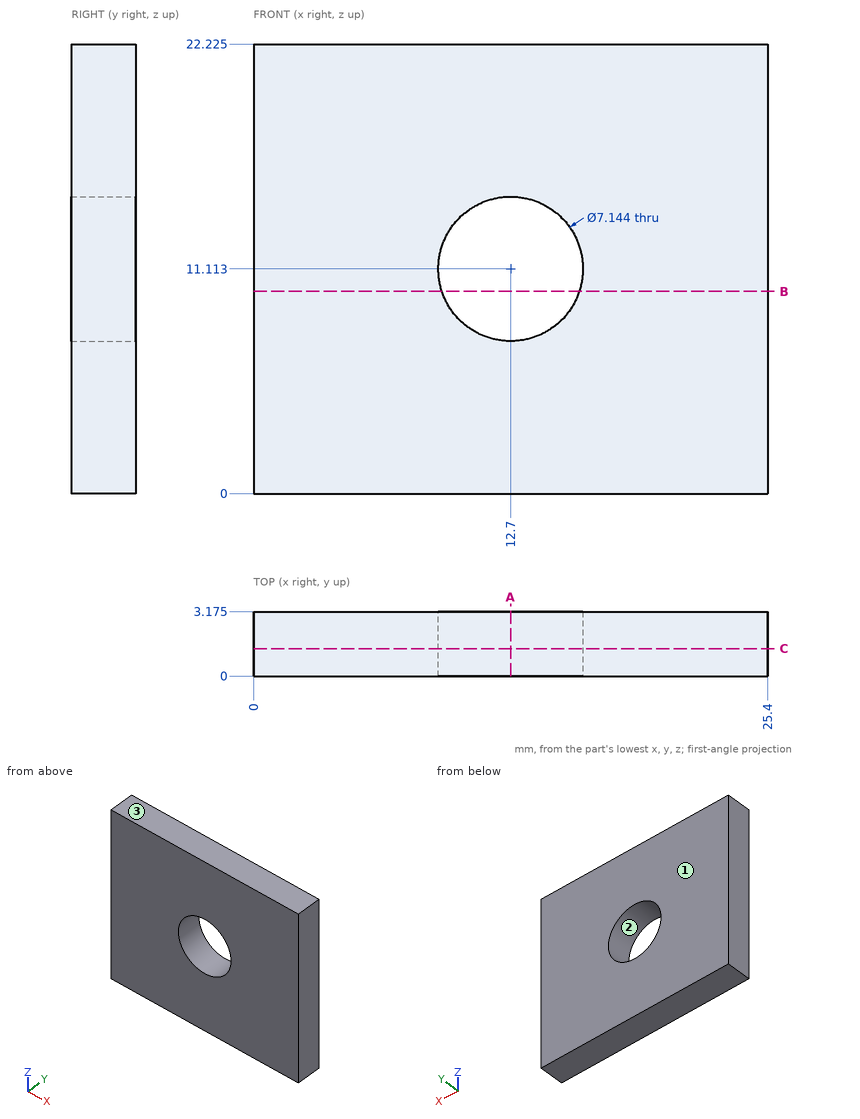
The drawing under review shows one solid part. Ordinate dimensions are in mm from its lowest x, y, z. Coordinates: 2 decimals unless noted, no trailing zeros. Write each loop counter-clockwise with the first axis right and the second up, starting at its lowest first coordinate (ties: lowest second). Pieces come first, ordered by that corner, then holes. Notation, with made-up numbers: (-24.75, 18) -> (-11.75, 18) arc R21 cw to (-11.75, 27) -> close; hole circle Ø6 at (-14.75, 29). An arc over 180 degrees is marked (long way). One line per item, written item: value. Start each with the question number.
Q1. Add section A-A, the plane x = 12.7. Give the boundary of the cut face in (y, z) (1 decimal).
Q2. Add section C-C, the plane y = 1.35. Give the boundary of the cut face in (x, z) (1 decimal).
Q3. Add section B-B, the plane z = 10. Give the boundary of the cut face in (x, y) (1 decimal).
Q4. The part is to be moulded in two halves that separate along Z. For the marked faces 1, 2 and 3, say which applies: +Z half, -Z half, draft (parallel to the pull), parting line (faces both ways), or undercut.
Q5. Clearance check with a flat-ended pin moving along its axis: P1, Ø3, axis at x = 8.5, z = 9, coming from the -Y side. State where the tip first meets the part, or that it passes through.
Q6. To check wall thickness, follow probe 1 along Z at (x, y) = (12.7, 1.7) (1 decimal); probe 2 along Z at (x, y) = (11, 3) (1 decimal); probe 3 along X at (y, z) = (0.7, 9). State the ranges of each line that lie inside material, in increasing order.
Response:
1. outline: (0, 0) -> (3.2, 0) -> (3.2, 7.5) -> (0, 7.5) -> close; (0, 14.7) -> (3.2, 14.7) -> (3.2, 22.2) -> (0, 22.2) -> close
2. outline: (0, 0) -> (25.4, 0) -> (25.4, 22.2) -> (0, 22.2) -> close; hole circle Ø7.1 at (12.7, 11.1)
3. outline: (0, 0) -> (9.3, 0) -> (9.3, 3.2) -> (0, 3.2) -> close; (16.1, 0) -> (25.4, 0) -> (25.4, 3.2) -> (16.1, 3.2) -> close
4. face 1: draft
4. face 2: undercut
4. face 3: +Z half
5. P1: y = 0
6. probe 1: 0 to 7.5, 14.7 to 22.2
6. probe 2: 0 to 8, 14.3 to 22.2
6. probe 3: 0 to 9.82, 15.58 to 25.4
